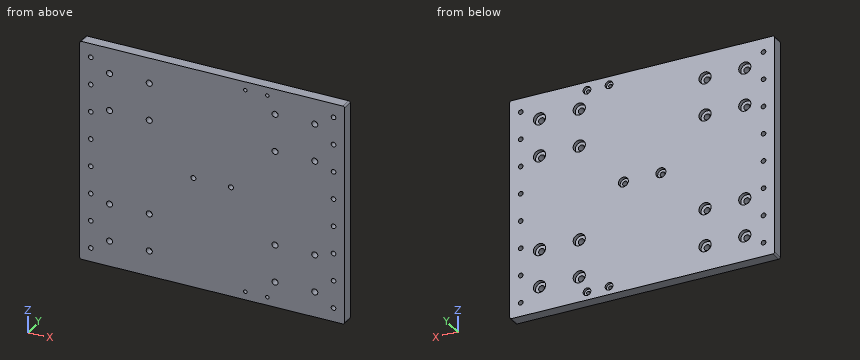
from build123d import *

# Parameters (mm, degrees)
SKETCH1_W                                        = 240
SKETCH1_H                                        = 200
BOSS_EXTRUDE1_DEPTH                              = 5
CBORE_FOR_M5_PAN_HEAD_MACHINE_SCREW1_D           = 5.5
CBORE_FOR_M5_PAN_HEAD_MACHINE_SCREW1_CBORE_D     = 11
CBORE_FOR_M5_PAN_HEAD_MACHINE_SCREW1_CBORE_DEPTH = 3.7
MIRROR2_COPY_1_D                                 = 5.5
MIRROR2_COPY_1_CBORE_D                           = 11
MIRROR2_COPY_1_CBORE_DEPTH                       = 3.7
CBORE_FOR_M4_PAN_HEAD_MACHINE_SCREW1_D           = 4.5
CBORE_FOR_M4_PAN_HEAD_MACHINE_SCREW1_CBORE_D     = 9
CBORE_FOR_M4_PAN_HEAD_MACHINE_SCREW1_CBORE_DEPTH = 3.1
M5X0_8_TAPPED_HOLE1_D                            = 4.2
FILLET1_R                                        = 1.5
LPATTERN2_COUNT                                  = 8
LPATTERN2_PITCH                                  = 25
CBORE_FOR_M3_PAN_HEAD_MACHINE_SCREW1_D           = 3.2
CBORE_FOR_M3_PAN_HEAD_MACHINE_SCREW1_CBORE_D     = 7
CBORE_FOR_M3_PAN_HEAD_MACHINE_SCREW1_CBORE_DEPTH = 2.4


with BuildPart() as part:
    # Sketch1 → Boss-Extrude1 (new body, symmetric)
    with BuildSketch(Plane(origin=(0, 0, 0), x_dir=(1, 0, 0), z_dir=(0, 1, 0))):
        Rectangle(SKETCH1_W, SKETCH1_H)
    extrude(amount=BOSS_EXTRUDE1_DEPTH, both=True)

    # CBORE for M5 Pan Head Machine Screw1 (through all)
    with Locations(Plane(origin=(66.92305649, 5, -81.969265096), x_dir=(-1, 0, 0), z_dir=(0, 1, 0))):
        with Locations((159.92305649, 158.969265096), (123.92305649, 158.969265096), (123.92305649, 124.969265096), (159.92305649, 124.969265096)):
            cbore_for_m5_pan_head_machine_screw1 = CounterBoreHole(CBORE_FOR_M5_PAN_HEAD_MACHINE_SCREW1_D / 2, CBORE_FOR_M5_PAN_HEAD_MACHINE_SCREW1_CBORE_D / 2, CBORE_FOR_M5_PAN_HEAD_MACHINE_SCREW1_CBORE_DEPTH)

    # Mirror1: CBORE for M5 Pan Head Machine Screw1 across plane
    add(cbore_for_m5_pan_head_machine_screw1.mirror(Plane(origin=(0, 0, 0), x_dir=(0, 0, 1), z_dir=(1, 0, 0))), mode=Mode.SUBTRACT)

    # Mirror2: CBORE for M5 Pan Head Machine Screw1 across plane
    add(cbore_for_m5_pan_head_machine_screw1.mirror(Plane.XY), mode=Mode.SUBTRACT)

    # Mirror2 copy 1 (through all)
    with Locations(Plane(origin=(-66.92305649, 5, 81.969265096), x_dir=(1, 0, 0), z_dir=(0, 1, 0))):
        with Locations((159.92305649, 158.969265096), (123.92305649, 158.969265096), (123.92305649, 124.969265096), (159.92305649, 124.969265096)):
            CounterBoreHole(MIRROR2_COPY_1_D / 2, MIRROR2_COPY_1_CBORE_D / 2, MIRROR2_COPY_1_CBORE_DEPTH)

    # CBORE for M4 Pan Head Machine Screw1 (through all)
    with Locations(Plane(origin=(-30.338508942, 5, -23.538498317), x_dir=(-1, 0, 0), z_dir=(0, 1, 0))):
        with Locations((-13.338508942, 23.538498317), (-47.338508942, 23.538498317)):
            CounterBoreHole(CBORE_FOR_M4_PAN_HEAD_MACHINE_SCREW1_D / 2, CBORE_FOR_M4_PAN_HEAD_MACHINE_SCREW1_CBORE_D / 2, CBORE_FOR_M4_PAN_HEAD_MACHINE_SCREW1_CBORE_DEPTH)

    # M5x0.8 Tapped Hole1 (through all)
    with Locations(Plane(origin=(0, 5, 0), x_dir=(1, 0, 0), z_dir=(0, 1, 0))):
        with Locations((-110, 87.5), (110, 87.5)):
            m5x0_8_tapped_hole1 = Hole(M5X0_8_TAPPED_HOLE1_D / 2)

    # Fillet1
    fillet1_edges = [part.edges().sort_by_distance(p)[0] for p in [
        (120, 0, 100),
        (-120, 0, 100),
        (-120, 0, -100),
        (120, 0, -100),
    ]]
    fillet(fillet1_edges, radius=FILLET1_R)

    # LPattern2: M5x0.8 Tapped Hole1 ×8
    with Locations(*[(0, 0, i * LPATTERN2_PITCH) for i in range(1, LPATTERN2_COUNT)]):
        add(m5x0_8_tapped_hole1, mode=Mode.SUBTRACT)

    # CBORE for M3 Pan Head Machine Screw1 (through all)
    with Locations(Plane(origin=(0, 5, 0), x_dir=(1, 0, 0), z_dir=(0, 1, 0))):
        with Locations((30, 92.5), (50, 92.5)):
            cbore_for_m3_pan_head_machine_screw1 = CounterBoreHole(CBORE_FOR_M3_PAN_HEAD_MACHINE_SCREW1_D / 2, CBORE_FOR_M3_PAN_HEAD_MACHINE_SCREW1_CBORE_D / 2, CBORE_FOR_M3_PAN_HEAD_MACHINE_SCREW1_CBORE_DEPTH)

    # Mirror3: CBORE for M3 Pan Head Machine Screw1 across plane
    add(cbore_for_m3_pan_head_machine_screw1.mirror(Plane.XY), mode=Mode.SUBTRACT)


solid = part.part
Read the model definition and answer for the solid it produces. Units are mm, in the model's axes. Coordinates: 2 decimals unless noted, no trailing zeros.
Q1. The part is cut by section A-A on z = -77. Give the number of separate pieces and of enclosed holes in the cut face, and give its area (3 significant figures).
Q2. Each of these flat-tipped pins is pushed along its axis until it touches: pin 1 Ø2.5 at (x, z) = (30, 92.5) entering from -Y; pin 2 Ø9 at (x, z) = (57.5, 43) entering from +Y. Where does it stop, or does it pass through?
Q3. Consider probe 1 along Z at (x, y) = (-57, -0.25); probe 2 along X at (y, z) = (-2.5, -43); probe 3 along X at (y, z) = (3.65, 77). Determine where each line is inside the solid, lowest interval first.
Results below:
1. separate pieces: 5
1. enclosed holes: 0
1. area: 2,100 mm2
2. pin 1: passes through
2. pin 2: stops at y = 1.3
3. probe 1: z = -100 to -79.75, -74.25 to -45.75, -40.25 to 40.25, 45.75 to 74.25, 79.75 to 100
3. probe 2: x = -120 to -95.75, -90.25 to -59.75, -54.25 to 54.25, 59.75 to 90.25, 95.75 to 120
3. probe 3: x = -120 to -98.5, -87.5 to -62.5, -51.5 to 51.5, 62.5 to 87.5, 98.5 to 120
